```python
from build123d import *

# Parameters (mm, degrees)
F1_DEPTH  = 3
F3_DEPTH  = 9
F5_DEPTH  = 9
F7_DEPTH  = 25
F9_DEPTH  = 25
F10_SIZE2 = 8.5069227294
F10_SIZE  = 1.5
F11_SIZE  = 1
F12_F1_R  = 1
F12_F2_R  = 1
F12_F3_R  = 1
F12_F4_R  = 1
F12_F5_R  = 1
F12_F6_R  = 1
F12_F7_R  = 1
F12_F8_R  = 1
F12_F9_R  = 1
F12_F10_R = 1
F12_F11_R = 1
F12_F12_R = 1
F12_F13_R = 1
F12_F14_R = 1
F12_F15_R = 1


with BuildPart() as f1:
    # F0 (on Top) → F1 (new body)
    with BuildSketch(Plane.XY):
        Polygon((0, 0), (-42, 42), (-42, 0), align=None)
    extrude(amount=F1_DEPTH)

    # F2 (on face) → F3 (join)
    with BuildSketch(Plane.XY.offset(3)):
        Polygon((-42, 37), (-42, 0), (-5, 0), (-5, 5), (-7, 7), (-35, 7), (-35, 35), (-37, 37), align=None)
    extrude(amount=F3_DEPTH)

    # F4 (on face) → F5 (cut)
    with BuildSketch(Plane.XY.offset(12)):
        Polygon((-39.55, 33.45), (-39.55, 2.45), (-8.55, 2.45), (-8.55, 4.55), (-37.45, 4.55), (-37.45, 33.45), align=None)
    extrude(amount=-F5_DEPTH, mode=Mode.SUBTRACT)

    # F6 (on face) → F7 (cut)
    with BuildSketch(Plane.XY.offset(3)):
        Polygon((-5, 5), (-5, 0), (0, 0), align=None)
    extrude(amount=-F7_DEPTH, mode=Mode.SUBTRACT)

    # F8 (on face) → F9 (cut)
    with BuildSketch(Plane.XY.offset(3)):
        Polygon((-42, 42), (-42, 37), (-37, 37), align=None)
    extrude(amount=-F9_DEPTH, mode=Mode.SUBTRACT)

    # F10
    f10_edges = [f1.edges().sort_by_distance(p)[0] for p in [
        (-23.5, 0, 12),
        (-5, 2.5, 12),
        (-6, 6, 12),
        (-21, 7, 12),
        (-35, 21, 12),
        (-36, 36, 12),
        (-39.5, 37, 12),
        (-42, 18.5, 12),
    ]]
    f10_side = f1.faces().sort_by_distance((-41.476741, 18.5, 12))[0]
    chamfer(f10_edges, length=F10_SIZE, length2=F10_SIZE2, reference=f10_side)

    # F11
    f11_edges = [f1.edges().sort_by_distance(p)[0] for p in [
        (-21, 21, 3),
    ]]
    chamfer(f11_edges, length=F11_SIZE)

    # F12: fillet of radius 1 on 17 edges, made by hand

    # F12_f1
    f12_f1_edges = [f1.edges().sort_by_distance(p)[0] for p in [
        (-7, 7, 2.5),
        (-7, 7, 3.2465386353),
    ]]
    fillet(f12_f1_edges, radius=F12_F1_R)

    # F12_f2
    f12_f2_edges = [f1.edges().sort_by_distance(p)[0] for p in [
        (-35, 35, 2.5),
        (-35, 35, 3.2465386353),
    ]]
    fillet(f12_f2_edges, radius=F12_F2_R)

    # F12_f3
    f12_f3_edges = [f1.edges().sort_by_distance(p)[0] for p in [
        (-5, 5, 1.7465386353),
    ]]
    fillet(f12_f3_edges, radius=F12_F3_R)

    # F12_f4
    f12_f4_edges = [f1.edges().sort_by_distance(p)[0] for p in [
        (-37, 37, 1.7465386353),
    ]]
    fillet(f12_f4_edges, radius=F12_F4_R)

    # F12_f5
    f12_f5_edges = [f1.edges().sort_by_distance(p)[0] for p in [
        (-5.7880602337, 4.6735747632, 7.962388947),
    ]]
    fillet(f12_f5_edges, radius=F12_F5_R)

    # F12_f6
    f12_f6_edges = [f1.edges().sort_by_distance(p)[0] for p in [
        (-7.3264252368, 6.2119397663, 7.962388947),
    ]]
    fillet(f12_f6_edges, radius=F12_F6_R)

    # F12_f7
    f12_f7_edges = [f1.edges().sort_by_distance(p)[0] for p in [
        (-5, 0, 1.7465386353),
    ]]
    fillet(f12_f7_edges, radius=F12_F7_R)

    # F12_f8
    f12_f8_edges = [f1.edges().sort_by_distance(p)[0] for p in [
        (-35.7880602337, 34.6735747632, 7.962388947),
    ]]
    fillet(f12_f8_edges, radius=F12_F8_R)

    # F12_f9
    f12_f9_edges = [f1.edges().sort_by_distance(p)[0] for p in [
        (-37.3264252368, 36.2119397663, 7.962388947),
    ]]
    fillet(f12_f9_edges, radius=F12_F9_R)

    # F12_f10
    f12_f10_edges = [f1.edges().sort_by_distance(p)[0] for p in [
        (-42, 37, 1.7465386353),
    ]]
    fillet(f12_f10_edges, radius=F12_F10_R)

    # F12_f11
    f12_f11_edges = [f1.edges().sort_by_distance(p)[0] for p in [
        (-35.75, 6.25, 7.7465386353),
    ]]
    fillet(f12_f11_edges, radius=F12_F11_R)

    # F12_f12
    f12_f12_edges = [f1.edges().sort_by_distance(p)[0] for p in [
        (-5.8964466094, 0.8964466094, 8.5770786288),
    ]]
    fillet(f12_f12_edges, radius=F12_F12_R)

    # F12_f13
    f12_f13_edges = [f1.edges().sort_by_distance(p)[0] for p in [
        (-42, 0, 1.7465386353),
    ]]
    fillet(f12_f13_edges, radius=F12_F13_R)

    # F12_f14
    f12_f14_edges = [f1.edges().sort_by_distance(p)[0] for p in [
        (-41.1035533906, 36.1035533906, 8.5770786288),
    ]]
    fillet(f12_f14_edges, radius=F12_F14_R)

    # F12_f15
    f12_f15_edges = [f1.edges().sort_by_distance(p)[0] for p in [
        (-41.1035533906, 0.8964466094, 8.5770786288),
    ]]
    fillet(f12_f15_edges, radius=F12_F15_R)


solid = f1.part
```
The listing builds one solid part. Answer for the finished solid, in the listing's coordinates (mm). A direction names the side the tool comes from. Give positions to 0.01 mm unless a question says otherwise; leave off trailing zeros. Write each loop counter-clockwise with the first axis right and the second up, starting at its lowest first coordinate (ties: lowest second). Pieces come first, ordered by that corner, then holes. Notation, with made-up numbers: M 58,-12 L 91,-12 A4 ccw 91,-7 Z; hole C -15.75,-40 d3. An arc over 180 degrees is marked long. Write each question's results on one line, items separated by ' | '.
Q1. Section A-A, the plane x = -39 is taken. Write down the section's boundary in (y, z), then the cut area to 3 significant figures.
Output values:
outline: M 0,0 L 37,0 L 37,3.49 L 35.5,12 L 33.45,12 L 33.45,3 L 2.45,3 L 2.45,12 L 1.5,12 L 0,3.49 Z | area: 152 mm2
Q2. Section B-B, the plane y = 17 is taken. Write down the section's boundary in (x, z), then the cut area to 3 significant figures.
Output values:
outline: M -42,0 L -17,0 L -17,2 L -18.41,3 L -35,3 L -35,3.49 L -36.5,12 L -37.45,12 L -37.45,3 L -39.55,3 L -39.55,12 L -40.5,12 L -42,3.49 Z | area: 106 mm2
Q3. For a pull along X with two mould halves and no side action, classify faces 1 (the flat face through (-28, 15, 3)), 2 (the flat face through (-36.4, 35.6, 6.7)), 3 (the cylindrical face through (-40.97, 35.96, 7.74)), 4 (the flat face through (-38, 11, 3)) as released by +X, released by -X, zero draft, split by the parting line, or undercut.
Output values:
face 1: zero draft | face 2: released by +X | face 3: released by -X | face 4: undercut
Q4. A tool of negligible diameter and unlimited length cuts with its end or side. For faces 5 (the flat face through (-23.75, 0.74, 7.69)), 6 (the flat face through (-21.26, 6.26, 7.69)), 7 (the flat face through (-23, 4.55, 8)), from which of +Z, -Z, +X, -X, +Y, -Y can it reach the whole face along a straight path? Write none if from no direction.
Output values:
face 5: +Z, +X, -X, -Y | face 6: +Z, +X, +Y | face 7: +Z
Q5. Consider L1, parallel to Z at x = -31, y = 29; L2, parallel to X at y = 30.5, z = 5; L3, parallel to X at y = 18, z = 3.75. Determine where each line is inside the solid, lowest interval first. Write a range as from..to.
Output values:
L1: 0..3 | L2: -41.73..-39.55, -37.45..-35.27 | L3: -41.95..-39.55, -37.45..-35.05
Q6. Flat-ended cylindrical pins translate along their axes: P1, Ø5, axis at y = 13.5, z = 3.5, coming from the +X side; P2, Ø1, axis at y = 3.5, z = 7.5, coming from the -X side; P3, Ø1, axis at x = -20.5, z = 9, coming from the -Y side; P4, Ø6, axis at x = -29, y = 7, coming from the -Z side. Find the tip coordinate at first contact, or state that the pin passes through.
Output values:
P1: x = -11.5 | P2: x = -41.38 | P3: y = 0.88 | P4: z = 0
Q7. Section C-C, the plane x = -13.5 is taken. Write down the section's boundary in (y, z), then the cut area to 3 significant figures.
Output values:
outline: M 0,0 L 13.5,0 L 13.5,2 L 12.09,3 L 7,3 L 7,3.49 L 5.5,12 L 4.55,12 L 4.55,3 L 2.45,3 L 2.45,12 L 1.5,12 L 0,3.49 Z | area: 71.1 mm2
